Work out the finished part from the listing and answer in its coordinate system (mm). Face numbers are marked on the shaded views. A direction names the side the tool comes from. Give positions to 0.01 mm unless a question says otherwise; leave off trailing zeros. Write each loop counter-clockwise with the first axis right and the second up, starting at its lowest first coordinate (ties: lowest second). Pieces come first, ordered by that corner, then holes. Notation, with made-up numbers: (-1.5, 24) - (23.5, 24) arc R30 cw to (23.5, 54) - close; hole circle Ø4 at (66, 72). An arc over 180 degrees is marked (long way). Write each question's results on one line, items separated by ' | '. Start each with the question number.
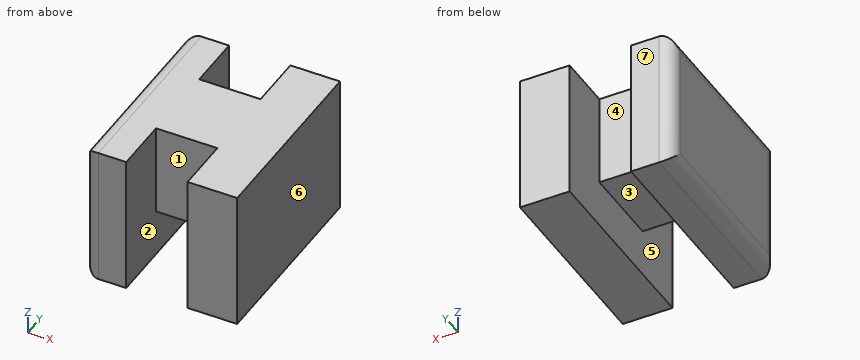
from build123d import *

# Parameters (mm, degrees)
SKETCH083_W  = 2.9
SKETCH083_H  = 3.305
PAD042_DEPTH = 2.2
SKETCH084_W  = 6.9
SKETCH084_H  = 5.01
PAD043_DEPTH = 1.78
SKETCH085_W  = 6.9
SKETCH085_H  = 5.01
PAD044_DEPTH = 1.5
FILLET006_R  = 0.5


with BuildPart() as part:
    # Sketch083 → Pad042 (new body)
    with BuildSketch(Plane.YZ):
        with Locations((-7.77, 12.9475)):
            Rectangle(SKETCH083_W, SKETCH083_H)
    extrude(amount=PAD042_DEPTH)

    # Sketch084 (on Face6 of Pad042) → Pad043 (join)
    with BuildSketch(Plane.YZ.offset(2.2)):
        with Locations((-7.77, 12.095)):
            Rectangle(SKETCH084_W, SKETCH084_H)
    extrude(amount=PAD043_DEPTH)

    # Sketch085 (on Face2 of Pad043) → Pad044 (join)
    with BuildSketch(Plane(origin=(0, 0, 0), x_dir=(0, 1, 0), z_dir=(-1, 0, 0))):
        with Locations((-7.77, -12.095)):
            Rectangle(SKETCH085_W, SKETCH085_H)
    extrude(amount=PAD044_DEPTH)

    # Fillet006
    fillet006_edges = [part.edges().sort_by_distance(p)[0] for p in [
        (-1.5, -11.22, 12.095),
        (-1.5, -7.77, 14.6),
        (-1.5, -4.32, 12.095),
        (-1.5, -7.77, 9.59),
    ]]
    fillet(fillet006_edges, radius=FILLET006_R)


with BuildPart() as part_1:
    # Body012 placement: moved
    add(part.part.moved(Location((-29.6, 0, 0))))


solid = part_1.part
Q1. Given pin 1 (1.1 mm diameter, centred on x = -29, y = -8, fed in from -Z) (3 decimals); pin 2 (0.7 mm diameter, centred on x = -28, z = 13.5, fed in from +Y), each flat-ended and moving along its own axis, determine where each tip first touches the part or whether it passes through.
Q2. A cutting plane is placed at D-D, the plane z = 12.6. Write down the section's boundary in (x, y), and give its area (3 significant figures).
Q3. A cutting plane is placed at C-C, the plane y = -6.5. Write down the section's boundary in (x, z) (3 decimals).
Q4. A cutting plane is placed at B-B, the plane y = -9.5. Write down the section's boundary in (x, z), and give its area (3 significant figures).
Q5. Consider L1, parallel to X at y = -8.75, z = 10.6; L2, parallel to Y at x = -28.7, z = 13.2; L3, parallel to Y at x = -30.65, z = 13. Determine where each line is inside the solid, lowest interval first.
Q6. A tool of negligible diameter and unlimited length cuts with its end or side. For the marked faces 1, 2, 3 and 4, from which of +Z, -Z, +X, -X, +Y, -Y can it reach the whole face along a straight path? Write none if from no direction.
Q7. The mould has two halves that part along X. Classify the marked faces 5, 6 and 7: pulls with the +X half, pulls with the -X half, needs draft (parallel to the pull), parting line crosses it, or undercut.
Q8. A cutting plane is placed at A-A, the plane z = 11.05. Write down the section's boundary in (x, y), and give its area (3 significant figures).
Result:
1) pin 1: stops at z = 11.295 | pin 2: stops at y = -6.32
2) outline: (-31.1, -10.72) arc R0.5 ccw to (-30.6, -11.22) - (-29.6, -11.22) - (-29.6, -9.22) - (-27.4, -9.22) - (-27.4, -11.22) - (-25.62, -11.22) - (-25.62, -4.32) - (-27.4, -4.32) - (-27.4, -6.32) - (-29.6, -6.32) - (-29.6, -4.32) - (-30.6, -4.32) arc R0.5 ccw to (-31.1, -4.82) - close | area: 28.9 mm2
3) outline: (-31.1, 10.09) arc R0.5 ccw to (-30.6, 9.59) - (-29.6, 9.59) - (-29.6, 11.295) - (-27.4, 11.295) - (-27.4, 9.59) - (-25.62, 9.59) - (-25.62, 14.6) - (-30.6, 14.6) arc R0.5 ccw to (-31.1, 14.1) - close
4) outline: (-31.1, 10.09) arc R0.5 ccw to (-30.6, 9.59) - (-29.6, 9.59) - (-29.6, 14.6) - (-30.6, 14.6) arc R0.5 ccw to (-31.1, 14.1) - close; (-27.4, 9.59) - (-25.62, 9.59) - (-25.62, 14.6) - (-27.4, 14.6) - close | area: 16.3 mm2
5) L1: x = -31.1 to -29.6, -27.4 to -25.62 | L2: y = -9.22 to -6.32 | L3: y = -11.22 to -4.32
6) face 1: +Z, -Z, -Y | face 2: -Z | face 3: -Z, +Y, -Y | face 4: +Z, -Z, +Y
7) face 5: undercut | face 6: pulls with the +X half | face 7: needs draft
8) outline: (-31.1, -10.72) arc R0.5 ccw to (-30.6, -11.22) - (-29.6, -11.22) - (-29.6, -4.32) - (-30.6, -4.32) arc R0.5 ccw to (-31.1, -4.82) - close; (-27.4, -11.22) - (-25.62, -11.22) - (-25.62, -4.32) - (-27.4, -4.32) - close | area: 22.5 mm2
